from build123d import *

# Parameters (mm, degrees)
F1_DEPTH       = 44.45
F3_D           = 6.35
F3_CSINK_D     = 10.16
F3_CSINK_ANGLE = 82
F4_T1_DEPTH    = 68.1485226281
F5_R           = 1.27


# Not quite as in the source:
# - a fillet or chamfer that OpenCascade refuses, or shapes differently, is made with other operations: its cross-section is extruded or revolved along the edge and cut away or added
# - a feature names something its author has since deleted; it is built from what else it names


with BuildPart() as f1:
    # F0 (on Top) → F1 (new body)
    with BuildSketch(Plane.XY):
        Polygon((0, 58.3955678842), (0, 0), (19.05, 0), (19.05, 25.4), align=None)
    extrude(amount=F1_DEPTH)

    # F3 (through all)
    with Locations(Plane(origin=(0, 0, 0), x_dir=(0, -1, 0), z_dir=(-1, 0, 0))):
        with Locations((-12.7, 22.225), (-38.1, 22.225)):
            CounterSinkHole(F3_D / 2, F3_CSINK_D / 2, counter_sink_angle=F3_CSINK_ANGLE)

    # F4: fillet of radius 1.27 on 1 edges, made by hand

    # F4_s2 → F4_t1 (cut)
    with BuildSketch(Plane.XY.offset(-11.849261314)):
        with BuildLine():
            ThreePointArc((0, 53.6558633586), (0.9412998127, 54.882589158), (2.3698522628, 54.2908633586))
            Line((2.3698522628, 54.2908633586), (0, 58.3955678842))
            Line((0, 58.3955678842), (0, 53.6558633586))
        make_face()
    extrude(amount=F4_T1_DEPTH, mode=Mode.SUBTRACT)

    # F5
    f5_edges = [f1.edges().sort_by_distance(p)[0] for p in [
        (0.9413, 54.882589, 44.45),
        (10.709926, 39.845432, 44.45),
        (19.05, 12.7, 44.45),
        (9.525, 0, 44.45),
        (0, 26.827932, 44.45),
        (0.9413, 54.882589, 0),
        (10.709926, 39.845432, 0),
        (19.05, 12.7, 0),
        (9.525, 0, 0),
        (0, 26.827932, 0),
        (0, 0, 22.225),
        (19.05, 0, 22.225),
    ]]
    fillet(f5_edges, radius=F5_R)


solid = f1.part
Build history of the part. All positions in model axes, mm. Give positions to 0.01 mm unless a question says otherwise; leave off trailing zeros. Loops run counter-clockwise (first coordinate to the right, second up) from the corner with the lowest first, then second, coordinate; pieces in that order, holes last. Notation, with made-up numbers: (13, 73.25) -> (21, 73.25) arc R5 cw to (21, 82.25) -> close; hole circle Ø10 at (39, -13.5). An arc over 180 degrees is marked (long way). Answer in a Markdown table with one row per item.
Item 1: Slice it at B-B on z = 30.5. Write the cut outline in (x, y), plus the area to 3 significant figures.
Findings below:
| item | result |
|---|---|
| outline | (0, 1.27) arc R1.27 ccw to (1.27, 0) -> (17.78, 0) arc R1.27 ccw to (19.05, 1.27) -> (19.05, 25.4) -> (2.37, 54.29) arc R1.27 ccw to (0, 53.66) -> close |
| area | 794 mm² |
Item 2: Slice it at C-C on z = 24.5. Give the number of separate pieces and of enclosed holes in the cut face, plus the area to 3 significant figures.
Findings below:
| item | result |
|---|---|
| separate pieces | 3 |
| enclosed holes | 0 |
| area | 647 mm² |
Item 3: Flat gauge pins, fed straight in: P1, Ø1, axis at y = 26, z = 32.5, coming from the +X side; P2, Ø1, axis at x = 3, z = 31.5, coming from the +Y side; P3, Ø8.5, axis at y = 12.7, z = 22.225, coming from the -X side. Where does each tip first touch, or does it go through?
Findings below:
| item | result |
|---|---|
| P1 | stops at x = 18.99 |
| P2 | stops at y = 54.07 |
| P3 | stops at x = 0.95 |
Item 4: Probe line 1 along Z through (x, y) = (6.5, 12.7); line 2 along Z through (x, y) = (11, 38.1); line 3 along Y through (x, z) = (11.25, 20). List the from-to ranges inside material, lowest first. Write a range as [from, to].
Findings below:
| item | result |
|---|---|
| line 1 | z = [0, 19.05], [25.4, 44.45] |
| line 2 | z = [0.18, 19.05], [25.4, 44.27] |
| line 3 | y = [0, 10.44], [14.96, 35.84] |
Item 5: Slice it at A-A on y = 12.7. Write the cut outline in (x, z) (3 decimals).
Findings below:
| item | result |
|---|---|
| outline | (0, 1.27) arc R1.27 ccw to (1.27, 0) -> (17.78, 0) arc R1.27 ccw to (19.05, 1.27) -> (19.05, 19.05) -> (2.191, 19.05) -> (0, 17.145) -> close; (0, 27.305) -> (2.191, 25.4) -> (19.05, 25.4) -> (19.05, 43.18) arc R1.27 ccw to (17.78, 44.45) -> (1.27, 44.45) arc R1.27 ccw to (0, 43.18) -> close |
Item 6: Mould opens along Y. For faces 1 (the cylindrical face through (10.496, 39.452, 0.362)), 2 (the cylindrical face through (10.74, 10.36, 24.37)), 3 (the cylindrical face through (0.362, 0.382, 22.518)) say: pulls with the +Y half, pulls with the -Y half, needs draft (parallel to the pull), parting line crosses it, or undercut.
Findings below:
| item | result |
|---|---|
| face 1 | pulls with the +Y half |
| face 2 | undercut |
| face 3 | pulls with the -Y half |
